The listing builds one solid part. Answer for the finished solid, in the listing's coordinates (mm). Face numbers are marked on the shaded views. A direction names the side the tool comes from. Coordinates: 2 decimals unless noted, no trailing zeros. Write each loop counter-clockwise with the first axis right and the second up, starting at its lowest first coordinate (ties: lowest second). Pieces come first, ordered by that corner, then holes.
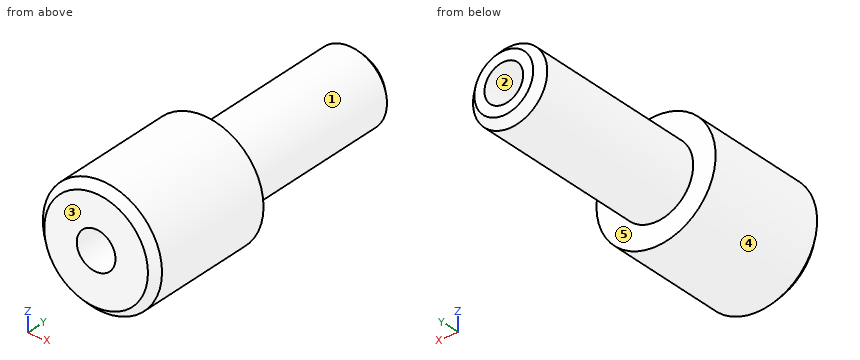
```python
from build123d import *

# Parameters (mm, degrees)
CHAMFER1_SIZE = 0.5


with BuildPart() as part:
    # Sketch1 → Revolve1 (revolve)
    with BuildSketch(Plane.XY):
        Polygon((1.25, 0), (1.25, 20.5), (2.4, 20.5), (2.4, 8.5), (3.85, 8.5), (3.85, 0), align=None)
    revolve(axis=Axis((0, 9.717567568, 0), (0, -1, 0)))

    # Chamfer1
    chamfer1_edges = [part.edges().sort_by_distance(p)[0] for p in [
        (-3.85, 0, 0),
        (-2.4, 20.5, 0),
    ]]
    chamfer(chamfer1_edges, length=CHAMFER1_SIZE)


solid = part.part
```
(1) Each of these flat-tipped pins is pushed along its axis until it touches: pin 1 (3 mm diameter, centred on x = 0, z = 0, fed in from -Y); pin 2 (1.5 mm diameter, centred on y = 11.5, z = 1, fed in from -X). Where does it stop, or does it pass through?
(2) Which of the six approach directions +Z, -Z, +X, -X, +Y, -Y give full straight-line access (tool end or side, diameter ignored) to the marked faces 4 and 5?
(3) Section C-C, the plane y = 19 is taken. Write down the section's boundary in (x, z), plus the area to 3 significant figures.
(4) Section B-B, the plane z = 0 is taken. Write down the section's boundary in (x, y), plus the area to 3 significant figures.
(5) For a pull along X with two mould halves and no side action, classify the marked faces 1, 2 and 3 as pulls with the +X half, pulls with the -X half, needs draft (parallel to the pull), parting line crosses it, or undercut.
(6) Find the intervals of material crossed by probe 1 along Z at (x, y) = (0, 15.25); probe 2 along Y at (x, z) = (-2, -1.5); probe 3 along Z at (x, y) = (0, 8), in increasing order.
(7) Section D-D, the plane y = 6.25 is taken. Write down the section's boundary in (x, z).
(8) Section A-A, the plane x = 0 is taken. Write down the section's boundary in (y, z).
Solution:
1. pin 1: stops at y = 0
1. pin 2: stops at x = -2.39
2. face 4: +Y, -Y
2. face 5: +Y
3. outline: circle Ø4.8 at (0, 0); hole circle Ø2.5 at (0, 0)
3. area: 13.2 mm2
4. outline: (-3.85, 0.5) - (-3.35, 0) - (-1.25, 0) - (-1.25, 20.5) - (-1.9, 20.5) - (-2.4, 20) - (-2.4, 8.5) - (-3.85, 8.5) - close; (1.25, 0) - (3.35, 0) - (3.85, 0.5) - (3.85, 8.5) - (2.4, 8.5) - (2.4, 20) - (1.9, 20.5) - (1.25, 20.5) - close
4. area: 71.3 mm2
5. face 1: parting line crosses it
5. face 2: undercut
5. face 3: needs draft
6. probe 1: z = -2.4 to -1.25, 1.25 to 2.4
6. probe 2: y = 0 to 8.5
6. probe 3: z = -3.85 to -1.25, 1.25 to 3.85
7. outline: circle Ø7.7 at (0, 0); hole circle Ø2.5 at (0, 0)
8. outline: (0, -3.35) - (0.5, -3.85) - (8.5, -3.85) - (8.5, -2.4) - (20, -2.4) - (20.5, -1.9) - (20.5, -1.25) - (0, -1.25) - close; (0, 1.25) - (20.5, 1.25) - (20.5, 1.9) - (20, 2.4) - (8.5, 2.4) - (8.5, 3.85) - (0.5, 3.85) - (0, 3.35) - close
